Could you check a few things on this model? Use its own coordinates, in mm. A direction names the side the tool comes from. Coordinates: 2 decimals unless noted, no trailing zeros. Order: outer loops, then holes, each group sorted by start corner. A loop starts at its lowest first (then second) coordinate and runs counter-clockwise, first axis right, second up. Notation, with made-up numbers: (36, -30) -> (85, -30) arc R37 ccw to (85, 7) -> close; hole circle Ø1 at (38.5, 51). An arc over 180 degrees is marked (long way). Use a Markdown table: item, result. Add a question column.
1) If I drill on L1, parallel to X at y = -46, z = 51.5; L2, parallel to X at y = -27.5, z = 62; L3, parallel to Z at x = -31, y = -40.5, over which ranges is the centre line in solid material (lowest first)? Write a range as [from, to].
2) Which directions (+Z, -Z, +X, -X, +Y, -Y) give clear straight access to the entire face, cutting with the end or side of a thin tool? Please do faces 1 (the flat face through (-28, -43.18, 31)), 2 (the flat face through (-60.138, -30.689, 63.877)), 3 (the cylindrical face through (-68.638, -46.937, 28.381)), 4 (the cylindrical face through (-27.644, -3.863, 38.906)), 5 (the flat face through (-46.028, -26, 57)).
3) Will these pins go through, and if not, where does the flat tip stop? pin 1 Ø5 at (x, y) = (-29, -29) entering from -Z; pin 2 Ø3.5 at (y, z) = (-17, 54.5) entering from +X.
4) If we section it at C-C (z = 56): Write out the boundary of the cut face in (x, y), plus the area to 3 significant figures.
5) If we section it at A-A (x = -49): Write out the boundary of the cut face in (y, z), plus the area to 3 significant figures.
6) Thinking about a two-plate mould opening in Y: for faces 6 (the flat face through (-66, 0, 33)), 7 (the flat face through (-47, -25, 32.558)), 8 (the cylindrical face through (-27.33, -46.937, 27.647)), which applies, +Y half, -Y half, draft (parallel to the pull), parting line (faces both ways), or undercut?
7) If we section it at D-D (x = -39.5): Write out the boundary of the cut face in (y, z), plus the area to 3 significant figures.
```python
from build123d import *

# Parameters (mm, degrees)
F1_DEPTH         = 50.8
F3_DEPTH         = 7.62
F3_COPIES_COUNT  = 2
F3_COPIES_PITCH  = 43.180422
F3_COPIES1_COUNT = 2
F3_COPIES1_PITCH = 57.645984
F5_DEPTH         = 7.62
F7_DEPTH         = 7.62
F9_DEPTH         = 7.62
F11_DEPTH        = 76.2
F13_DEPTH        = 76.2
F14_W            = 45.0653012376
F14_H            = 10.795
F15_DEPTH        = 3.81
F17_DEPTH        = 7.62
F19_DEPTH        = 7.62
F21_DEPTH        = 7.62
F23_DEPTH        = 7.62


# Not quite as in the source:
# - a pattern or mirror of a feature is missing from the dataset's text; its kind, count and spacing are read off the source's solid


with BuildPart() as f1:
    # F0 (on Front) → F1 (new body)
    with BuildSketch(Plane.XZ):
        Polygon((-75.7135227323, 45.2577668846), (-75.7135227323, 32.5577668846), (-18.04306696, 32.5577668846), (-18.04306696, 34.4673171639), (-18.04306696, 50.3806362459), (-24.2752695117, 64.5659697758), (-59.8352695117, 64.5659697758), (-66.0674720634, 50.3806362459), align=None)
    extrude(amount=F1_DEPTH)

    # F2 (on face) → F3 (cut)
    with BuildSketch(Plane.XZ.offset(50.8)):
        with BuildLine():
            Line((-72.3248315811, 32.5577668846), (-59.6248315811, 32.5577668846))
            ThreePointArc((-59.6248315811, 32.5577668846), (-65.9748315811, 38.9077668846), (-72.3248315811, 32.5577668846))
        make_face()
    f3 = extrude(amount=-F3_DEPTH, mode=Mode.SUBTRACT)

    # F3_copies: F3 ×2
    with Locations(*[Vector(-0.004422337, 0.9999902214, 0) * (i * F3_COPIES_PITCH) for i in range(1, F3_COPIES_COUNT)]):
        add(f3, mode=Mode.SUBTRACT)

    # F3_copies1: F3 ×2
    with Locations(*[Vector(0.662508063, 0.749054782, 0) * (i * F3_COPIES1_PITCH) for i in range(1, F3_COPIES1_COUNT)]):
        add(f3, mode=Mode.SUBTRACT)

    # F4 (on face) → F5 (join)
    with BuildSketch(Plane.XZ.offset(43.18)):
        with BuildLine():
            Line((-70.9278315811, 32.5577668846), (-61.0218315811, 32.5577668846))
            ThreePointArc((-61.0218315811, 32.5577668846), (-65.9748315811, 37.5107668846), (-70.9278315811, 32.5577668846))
        make_face()
        with BuildLine():
            ThreePointArc((-70.9278315811, 32.5577668846), (-65.9748315811, 27.6047668846), (-61.0218315811, 32.5577668846))
            Line((-61.0218315811, 32.5577668846), (-70.9278315811, 32.5577668846))
        make_face()
    extrude(amount=F5_DEPTH)

    # F6 (on face) → F7 (cut)
    with BuildSketch(Plane.XZ.offset(50.8)):
        with BuildLine():
            Line((-34.3248570174, 32.5577668846), (-21.6248570174, 32.5577668846))
            ThreePointArc((-21.6248570174, 32.5577668846), (-27.9748570174, 38.9077668846), (-34.3248570174, 32.5577668846))
        make_face()
    extrude(amount=-F7_DEPTH, mode=Mode.SUBTRACT)

    # F8 (on face) → F9 (join)
    with BuildSketch(Plane.XZ.offset(43.18)):
        with BuildLine():
            Line((-32.9278570174, 32.5577668846), (-23.0218570174, 32.5577668846))
            ThreePointArc((-23.0218570174, 32.5577668846), (-27.9748570174, 37.5107668846), (-32.9278570174, 32.5577668846))
        make_face()
        with BuildLine():
            ThreePointArc((-32.9278570174, 32.5577668846), (-27.9748570174, 27.6047668846), (-23.0218570174, 32.5577668846))
            Line((-23.0218570174, 32.5577668846), (-32.9278570174, 32.5577668846))
        make_face()
    extrude(amount=F9_DEPTH)

    # F10 (on face) → F11 (cut)
    with BuildSketch(Plane.XZ.offset(50.8)):
        Polygon((-46.0276552343, 62.4638214125), (-57.3104978095, 62.4638214125), (-62.5376552343, 50.8894175291), (-46.0276552343, 50.8894175291), align=None)
    extrude(amount=-F11_DEPTH, mode=Mode.SUBTRACT)

    # F12 (on face) → F13 (cut)
    with BuildSketch(Plane.XZ.offset(50.8)):
        Polygon((-26.6381744295, 62.4638214125), (-42.0552695117, 62.4638214125), (-42.0552695117, 50.8814214125), (-22.2462173551, 50.8814214125), align=None)
    extrude(amount=-F13_DEPTH, mode=Mode.SUBTRACT)

    # F14 (on face) → F15 (cut)
    with BuildSketch(Plane(origin=(-73.9314589089, 0, 32.4811415881), x_dir=(0, -1, 0), z_dir=(-0.9155372099, 0, 0.4022332872))):
        with Locations((24.9195831129, 27.1725985175)):
            Rectangle(F14_W, F14_H)
    extrude(amount=-F15_DEPTH, mode=Mode.SUBTRACT)

    # F16 (on face) → F17 (cut)
    with BuildSketch(Plane(origin=(0, 0, 0), x_dir=(-1, 0, 0), z_dir=(0, 1, 0))):
        with BuildLine():
            ThreePointArc((21.433902362, 32.5577668846), (27.783902362, 26.2077668846), (34.133902362, 32.5577668846))
            ThreePointArc((34.133902362, 32.5577668846), (27.783902362, 38.9077668846), (21.433902362, 32.5577668846))
        make_face()
    extrude(amount=-F17_DEPTH, mode=Mode.SUBTRACT)

    # F18 (on face) → F19 (join)
    with BuildSketch(Plane(origin=(0, -7.62, 0), x_dir=(-1, 0, 0), z_dir=(0, 1, 0))):
        with BuildLine():
            Line((22.830902362, 32.5577668846), (32.736902362, 32.5577668846))
            ThreePointArc((32.736902362, 32.5577668846), (27.783902362, 37.5107668846), (22.830902362, 32.5577668846))
        make_face()
        with BuildLine():
            ThreePointArc((22.830902362, 32.5577668846), (27.783902362, 27.6047668846), (32.736902362, 32.5577668846))
            Line((32.736902362, 32.5577668846), (22.830902362, 32.5577668846))
        make_face()
    extrude(amount=F19_DEPTH)

    # F20 (on face) → F21 (cut)
    with BuildSketch(Plane(origin=(0, 0, 0), x_dir=(-1, 0, 0), z_dir=(0, 1, 0))):
        with BuildLine():
            ThreePointArc((59.8157899618, 32.5577668846), (66.1657899618, 26.2077668846), (72.5157899618, 32.5577668846))
            ThreePointArc((72.5157899618, 32.5577668846), (66.1657899618, 38.9077668846), (59.8157899618, 32.5577668846))
        make_face()
    extrude(amount=-F21_DEPTH, mode=Mode.SUBTRACT)

    # F22 (on face) → F23 (join)
    with BuildSketch(Plane(origin=(0, -7.62, 0), x_dir=(-1, 0, 0), z_dir=(0, 1, 0))):
        with BuildLine():
            ThreePointArc((61.2127899618, 32.5577668846), (66.1657899618, 27.6047668846), (71.1187899618, 32.5577668846))
            Line((71.1187899618, 32.5577668846), (61.2127899618, 32.5577668846))
        make_face()
        with BuildLine():
            Line((61.2127899618, 32.5577668846), (71.1187899618, 32.5577668846))
            ThreePointArc((71.1187899618, 32.5577668846), (66.1657899618, 37.5107668846), (61.2127899618, 32.5577668846))
        make_face()
    extrude(amount=F23_DEPTH)


solid = f1.part
```
Answer sheet:
| question | item | result |
|---|---|---|
| 1 | L1 | [-65.58, -63.09], [-46.03, -42.06], [-22.48, -18.53] |
| 1 | L2 | [-60.15, -57.52], [-46.03, -42.06], [-26.46, -23.15] |
| 1 | L3 | [32.56, 50.88], [62.46, 64.57] |
| 2 | face 1 | -Z, +X, -X |
| 2 | face 2 | +Z, -X, +Y, -Y |
| 2 | face 3 | -Y |
| 2 | face 4 | +Y |
| 2 | face 5 | +Y, -Y |
| 3 | pin 1 | z = 32.56 |
| 3 | pin 2 | x = -19.08 |
| 4 | outline | (-63.6, -50.8) -> (-60.23, -50.8) -> (-60.23, -47.45) -> (-63.6, -47.45) -> close; (-63.6, -2.39) -> (-60.23, -2.39) -> (-60.23, 0) -> (-63.6, 0) -> close; (-46.03, -50.8) -> (-42.06, -50.8) -> (-42.06, 0) -> (-46.03, 0) -> close; (-24.19, -50.8) -> (-20.51, -50.8) -> (-20.51, 0) -> (-24.19, 0) -> close |
| 4 | area | 408 mm2 |
| 5 | outline | (-50.8, 32.56) -> (0, 32.56) -> (0, 50.89) -> (-50.8, 50.89) -> close; (-50.8, 62.46) -> (0, 62.46) -> (0, 64.57) -> (-50.8, 64.57) -> close |
| 5 | area | 1,040 mm2 |
| 6 | face 6 | +Y half |
| 6 | face 7 | undercut |
| 6 | face 8 | draft |
| 7 | outline | (-50.8, 32.56) -> (0, 32.56) -> (0, 50.88) -> (-50.8, 50.88) -> close; (-50.8, 62.46) -> (0, 62.46) -> (0, 64.57) -> (-50.8, 64.57) -> close |
| 7 | area | 1,040 mm2 |
